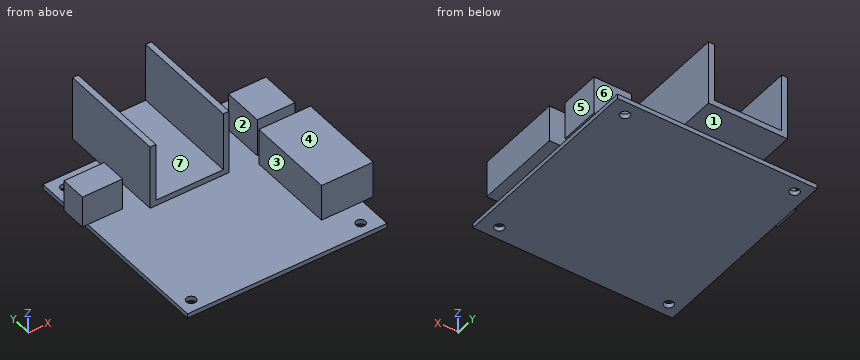
from build123d import *

# Parameters (mm, degrees)
SKETCH_W     = 69.52
SKETCH_H     = 70.79
SKETCH_R     = 1.65
PAD_DEPTH    = 1.6
SKETCH001_W  = 18
SKETCH001_H  = 30.7
PAD001_DEPTH = 12.75
SKETCH002_W  = 13.1
SKETCH002_H  = 14.1
PAD002_DEPTH = 13.2
SKETCH003_W  = 14
SKETCH003_H  = 9
PAD003_DEPTH = 11
SKETCH004_W  = 27.5
SKETCH004_H  = 38
PAD004_DEPTH = 22.55
SKETCH005_W  = 23.5
SKETCH005_H  = 23.222077
POCKET_DEPTH = 38


with BuildPart() as part:
    # Sketch → Pad (new body)
    with BuildSketch(Plane.XY):
        Rectangle(SKETCH_W, SKETCH_H)
        with Locations((-30.315, 30.645)):
            Circle(SKETCH_R, mode=Mode.SUBTRACT)
        with Locations((28.74, 30.645)):
            Circle(SKETCH_R, mode=Mode.SUBTRACT)
        with Locations((-30.315, -30.95)):
            Circle(SKETCH_R, mode=Mode.SUBTRACT)
        with Locations((28.74, -30.95)):
            Circle(SKETCH_R, mode=Mode.SUBTRACT)
    extrude(amount=PAD_DEPTH)

    # Sketch001 (on Face10 of Pad) → Pad001 (join)
    with BuildSketch(Plane.XY.offset(1.6)):
        with Locations((29.46, -8.09)):
            Rectangle(SKETCH001_W, SKETCH001_H)
    extrude(amount=PAD001_DEPTH)

    # Sketch002 (on Face5 of Pad001) → Pad002 (join)
    with BuildSketch(Plane.XY.offset(1.6)):
        with Locations((28.81, 17.6275)):
            Rectangle(SKETCH002_W, SKETCH002_H)
    extrude(amount=PAD002_DEPTH)

    # Sketch003 (on Face5 of Pad002) → Pad003 (join)
    with BuildSketch(Plane.XY.offset(1.6)):
        with Locations((-29.64, 17.945)):
            Rectangle(SKETCH003_W, SKETCH003_H)
    extrude(amount=PAD003_DEPTH)

    # Sketch004 (on Face5 of Pad003) → Pad004 (join)
    with BuildSketch(Plane.XY.offset(1.6)):
        with Locations((-2.375, 28.095)):
            Rectangle(SKETCH004_W, SKETCH004_H)
    extrude(amount=PAD004_DEPTH)

    # Sketch005 (on Face27 of Pad004) → Pocket (cut)
    with BuildSketch(Plane(origin=(0, 47.095, 0), x_dir=(-1, 0, 0), z_dir=(0, 1, 0))):
        with Locations((2.375, 15.211039)):
            Rectangle(SKETCH005_W, SKETCH005_H)
    extrude(amount=-POCKET_DEPTH, mode=Mode.SUBTRACT)


solid = part.part
Input: part model. Units: mm. Frame: model coordinates. Face numbers are marked on the shaded views. A direction names the side the tool comes from. Round coordinates to 2 decimals unless told otherwise and drop trailing zeros. Loops run counter-clockwise (first coordinate to the right, second up) from the corner with the lowest first, then second, coordinate; pieces in that order, holes last. Notation, with made-up numbers: (-23.75, -4.5) -> (-14.75, -4.5) arc R30 cw to (-14.75, 23.5) -> close; hole circle Ø4 at (-9, -20.75). An arc over 180 degrees is marked (long way). Answer as a JSON object with one key per item and string values. Group by question number.
1) Pin query (flat end, axial travel): pin 1 (6 mm diameter, centred on y = 35.5, z = 6.5, fed in from +X) (3 decimals); pin 2 (1.8 mm diameter, centred on x = 0, z = 0.5, fed in from +Y) (3 decimals); pin 3 (4.5 mm diameter, centred on x = -28, y = 17, fed in from +Z). Return the tip coordinate at first contact, or that it passes through.
2) Section query A-A on z = 19.25. Output: boundary loops of the cut face in (x, y) (3 decimals).
3) Draft query along X for the marked faces 1, 2 and 3. Return one class per face: +X half, -X half, draft (parallel to the pull), parting line (faces both ways), or undercut.
4) Section query B-B on y = -30.95. Output: boundary loops of the cut face in (x, z) (3 decimals), plus the area to 3 significant figures.
5) Section query D-D on x = 28.74. State how many separate pieces and enclosed holes the cut face has, plus the area to 3 significant figures.
6) Ray query, L1, parallel to X at y = 11.5, z = 7.5 (3 decimals); L2, parallel to Y at x = 28.74, z = 1.1 (3 decimals); L3, parallel to X at y = 41, z = 4 (3 decimals). Return the intervals inside material, ascending.
7) Section query C-C on z = 7.25. Output: boundary loops of the cut face in (x, y) (1 decimal).
8) Reachability of the marked faces 4, 5, 6 and 7 from +Z, -Z, +X, -X, +Y, -Y: full face, straight path, thin tool, end or side. Return the list, or none.
Reply:
{
 "1": {"pin 1": "stops at x = 11.375", "pin 2": "stops at y = 35.395", "pin 3": "stops at z = 12.6"},
 "2": {"outline": "(-16.125, 9.095) -> (-14.125, 9.095) -> (-14.125, 47.095) -> (-16.125, 47.095) -> close; (9.375, 9.095) -> (11.375, 9.095) -> (11.375, 47.095) -> (9.375, 47.095) -> close"},
 "3": {"face 1": "draft", "face 2": "undercut", "face 3": "-X half"},
 "4": {"outline": "(-34.76, 0) -> (-31.965, 0) -> (-31.965, 1.6) -> (-34.76, 1.6) -> close; (-28.665, 0) -> (27.09, 0) -> (27.09, 1.6) -> (-28.665, 1.6) -> close; (30.39, 0) -> (34.76, 0) -> (34.76, 1.6) -> (30.39, 1.6) -> close", "area": "101 mm2"},
 "5": {"separate pieces": "3", "enclosed holes": "0", "area": "680 mm2"},
 "6": {"L1": "x = -16.125 to -14.125, 9.375 to 11.375, 22.26 to 35.36", "L2": "y = -35.395 to -32.6, -29.3 to 28.995, 32.295 to 35.395", "L3": "x = -16.125 to -14.125, 9.375 to 11.375"},
 "7": {"outline": "(-36.6, 13.4) -> (-22.6, 13.4) -> (-22.6, 22.4) -> (-36.6, 22.4) -> close; (-16.1, 9.1) -> (-14.1, 9.1) -> (-14.1, 47.1) -> (-16.1, 47.1) -> close; (9.4, 9.1) -> (11.4, 9.1) -> (11.4, 47.1) -> (9.4, 47.1) -> close; (20.5, -23.4) -> (38.5, -23.4) -> (38.5, 7.3) -> (20.5, 7.3) -> close; (22.3, 10.6) -> (35.4, 10.6) -> (35.4, 24.7) -> (22.3, 24.7) -> close"},
 "8": {"face 4": "+Z, +X, -X, -Y", "face 5": "+Z, -Z, +X, +Y", "face 6": "+Z, +X, +Y", "face 7": "+Z, +Y, -Y"}
}
